```python
from build123d import *

# Parameters (mm, degrees)
BOSS_EXTRU_1_DEPTH = 3


with BuildPart() as part:
    # Esquisse1 → Boss.-Extru.1 (new body)
    with BuildSketch(Plane.XY):
        with BuildLine():
            Line((0, 20), (0, 0))
            Line((0, 0), (20, 0))
            ThreePointArc((20, 0), (26.157688743, 3.708286934), (33.228756555, 5))
            Line((33.228756555, 5), (70, 5))
            Line((70, 5), (70, 15))
            Line((70, 15), (33.228756555, 15))
            ThreePointArc((33.228756555, 15), (26.157688743, 16.291713066), (20, 20))
            Line((20, 20), (0, 20))
        make_face()
    boss_extru_1 = extrude(amount=BOSS_EXTRU_1_DEPTH)

    # Symétrie7: Boss.-Extru.1 across plane
    add(boss_extru_1.mirror(Plane(origin=(70, 15, 3), x_dir=(0, 0, 1), z_dir=(-1, 0, 0))))


solid = part.part
```
Can you work these out from the model? Positions are in its coordinate system, mm. A direction names the side the tool comes from. Coordinates: 2 decimals unless noted, no trailing zeros. Write each loop counter-clockwise with the first axis right and the second up, starting at its lowest first coordinate (ties: lowest second). Pieces come first, ordered by that corner, then holes. Notation, with made-up numbers: M 18,-34.5 L 26,-34.5 A24 ccw 26,-22.5 Z; hole C -1.75,-29.75 d1. An arc over 180 degrees is marked long. Write item = value, one per line. Start each with the question number.
Q1. On a 3-axis mill with a long thin cutter (end or side, diameter ignored), from which of +Z, -Z, +X, -X, +Y, -Y can I reach the whole of each face in a straight line? I mean faces 1 (the face through (10, 20, 1)), 2 (the face through (113.748, 16.256, 1.479)), 3 (the face through (71, 5, 1)). Say none if no direction works.
Q2. If I drill on L1, parallel to Y at x = 83.5, z = 0.85; L2, parallel to X at y = 2.25, z = 1.9; L3, parallel to Y at x = 119, z = 1.8, over which ranges is the centre line in solid material (lowest first)? Write a range as [from, to].
Q3. Thinking about a two-plate mould opening in X: for faces 4 (the face through (26.06, 3.67, 1.48)), 5 (the face through (26.252, 16.256, 1.479)), 6 (the face through (130, 20, 1)), 7 (the face through (140, 10, 1)), which applies, released by +X, released by -X, zero draft, split by the parting line, or undercut?
Q4. If we section it at B-B, the plane y = 16.75: Write out the boundary of the cut face in (x, z), then the cut area to 3 significant figures.
Q5. I'm going to push flat-ended pins straight in: pin 1 (0.9 mm diameter, centred on x = 69, z = 1.5, fed in from -Y); pin 2 (0.9 mm diameter, centred on x = 79.5, z = 1.5, fed in from +Y); pin 3 (1 mm diameter, centred on x = 55.5, y = 17, fed in from +Z). Where does each tip first touch, or does it pass through?
Q6. If we section it at A-A, the plane z = 2.4: Write out the boundary of the cut face in (x, y).
Q7. If we section it at D-D, the plane y = 2.5: Write out the boundary of the cut face in (x, z).
Q8. If we section it at C-C, the plane x = 109.5: Write out the boundary of the cut face in (y, z).
Check sheet entries:
q1.face_1 = +Z, -Z, +X, -X, +Y
q1.face_2 = +Z, -Z, +Y
q1.face_3 = +Z, -Z, -Y
q2.L1 = [5, 15]
q2.L2 = [0, 23.11], [116.89, 140]
q2.L3 = [0.83, 19.17]
q3.face_4 = undercut
q3.face_5 = undercut
q3.face_6 = zero draft
q3.face_7 = released by +X
q4.outline = M 0,0 L 25.05,0 L 25.05,3 L 0,3 Z; M 114.95,0 L 140,0 L 140,3 L 114.95,3 Z
q4.area = 150 mm²
q5.pin_1 = 5
q5.pin_2 = 15
q5.pin_3 = through
q6.outline = M 0,0 L 20,0 A20 cw 33.23,5 L 106.77,5 A20 cw 120,0 L 140,0 L 140,20 L 120,20 A20 cw 106.77,15 L 33.23,15 A20 cw 20,20 L 0,20 Z
q7.outline = M 0,0 L 23.55,0 L 23.55,3 L 0,3 Z; M 116.45,0 L 140,0 L 140,3 L 116.45,3 Z
q8.outline = M 4.81,0 L 15.19,0 L 15.19,3 L 4.81,3 Z
